Geometry check sheet. Reference: the model listing, model coordinates, mm. Face numbers are marked on the shaded views. A direction names the side the tool comes from. Round coordinates to 2 decimals unless told otherwise and drop trailing zeros. Write each loop counter-clockwise with the first axis right and the second up, starting at its lowest first coordinate (ties: lowest second). Pieces come first, ordered by that corner, then holes.
Item 1: Cross-section at C-C (z = 5.5). Enter the section's corners in (x, y), then the cut area to 3 significant figures.
Item 2: Access from +Z, -Z, +X, -X, +Y, -Y to the whole of each face (thin tool, end or side, straight path). Record for the marked faces 1 and 2.
Item 3: Cross-section at D-D (y = 9.25). Enter the section's corners in (x, z), then the cut area to 3 significant figures.
Item 4: Cross-section at A-A (x = 7.5). Enter the section's corners in (y, z).
Item 5: Draft check along X on the marked faces 3, 4 and 5. Enter one of: pulls with the +X half, pulls with the -X half, needs draft (parallel to the pull), parting line crosses it, or undercut.
Item 6: Scan lines: probe 1 along X at (y, z) = (-4, 0.75); probe 2 along X at (y, z) = (9.25, 8.5). Record each from-to range of solid material in increasing order.
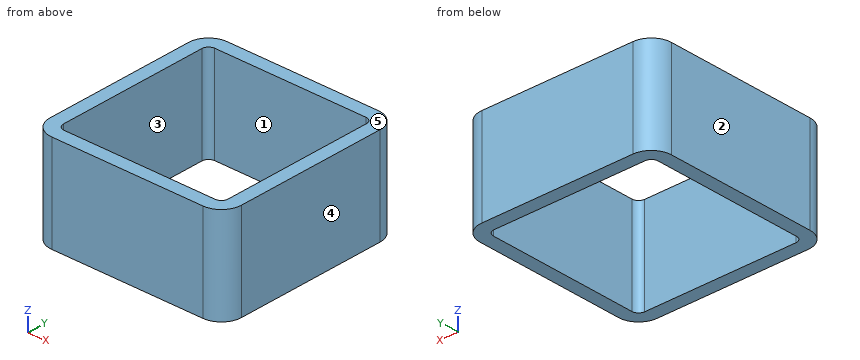
from build123d import *

# Parameters (mm, degrees)
F0_W     = 20
F0_H     = 20
F0_W_2   = 17.2
F0_H_2   = 17.2
F1_DEPTH = 10
F2_R     = 2.1
F3_R     = 2.1
F4_R     = 0.7
F5_R     = 0.7
F6_R     = 0.7
F7_R     = 0.7


with BuildPart() as f1:
    # F0 (on Top) → F1 (new body)
    with BuildSketch(Plane.XY):
        Rectangle(F0_W, F0_H)
        Rectangle(F0_W_2, F0_H_2, mode=Mode.SUBTRACT)
    extrude(amount=F1_DEPTH)

    # F2
    f2_edges = [f1.edges().sort_by_distance(p)[0] for p in [
        (-10, -10, 5),
        (10, -10, 5),
        (10, 10, 5),
    ]]
    fillet(f2_edges, radius=F2_R)

    # F3
    f3_edges = [f1.edges().sort_by_distance(p)[0] for p in [
        (-10, 10, 5),
    ]]
    fillet(f3_edges, radius=F3_R)

    # F4
    f4_edges = [f1.edges().sort_by_distance(p)[0] for p in [
        (-8.6, 8.6, 5),
    ]]
    fillet(f4_edges, radius=F4_R)

    # F5
    f5_edges = [f1.edges().sort_by_distance(p)[0] for p in [
        (-8.6, -8.6, 5),
    ]]
    fillet(f5_edges, radius=F5_R)

    # F6
    f6_edges = [f1.edges().sort_by_distance(p)[0] for p in [
        (8.6, -8.6, 5),
    ]]
    fillet(f6_edges, radius=F6_R)

    # F7
    f7_edges = [f1.edges().sort_by_distance(p)[0] for p in [
        (8.6, 8.6, 5),
    ]]
    fillet(f7_edges, radius=F7_R)


solid = f1.part
Resolved:
1. outline: (-10, -7.9) arc R2.1 ccw to (-7.9, -10) - (7.9, -10) arc R2.1 ccw to (10, -7.9) - (10, 7.9) arc R2.1 ccw to (7.9, 10) - (-7.9, 10) arc R2.1 ccw to (-10, 7.9) - close; hole (-8.6, -7.9) arc R0.7 ccw to (-7.9, -8.6) - (7.9, -8.6) arc R0.7 ccw to (8.6, -7.9) - (8.6, 7.9) arc R0.7 ccw to (7.9, 8.6) - (-7.9, 8.6) arc R0.7 ccw to (-8.6, 7.9) - close
1. area: 101 mm2
2. face 1: +Z, -Z
2. face 2: +Z, -Z, -X, +Y, -Y
3. outline: (-9.51, 0) - (9.51, 0) - (9.51, 10) - (-9.51, 10) - close
3. area: 190 mm2
4. outline: (-10, 0) - (-8.6, 0) - (-8.6, 10) - (-10, 10) - close; (8.6, 0) - (10, 0) - (10, 10) - (8.6, 10) - close
5. face 3: undercut
5. face 4: pulls with the +X half
5. face 5: needs draft
6. probe 1: x = -10 to -8.6, 8.6 to 10
6. probe 2: x = -9.51 to 9.51
